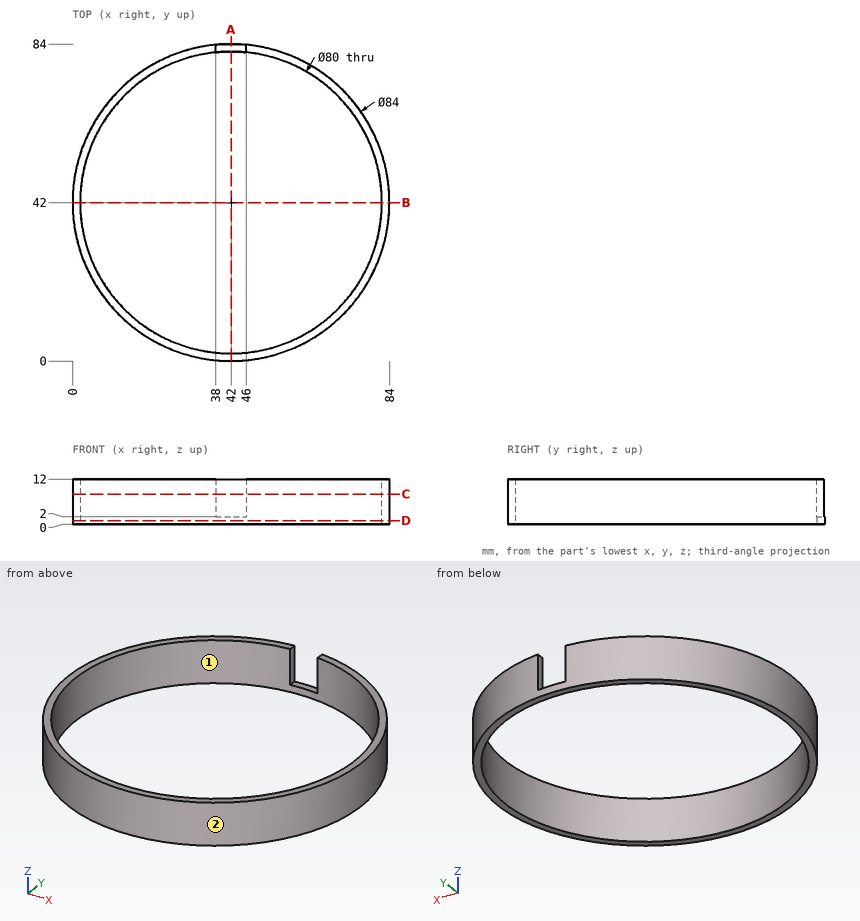
Drawing for the job (mm, zero at the part's lowest x, y, z). Give positions to 0.01 mm unless a question says otherwise; leave off trailing zeros. Order: outer loops, then holes, each group sorted by start corner. A loop starts at its lowest first (then second) coordinate and runs counter-clockwise, first axis right, second up. Notation, with made-up numbers: M -37.75,30.25 L -14.75,30.25 A17 cw -14.75,40.25 Z; hole C 56,-16.75 d10. An arc over 180 degrees is marked long. Write item = value, one per line. Start each with the question number.
(1) Slice it at A-A on x = 42. Write the cut outline in (y, z), plus the area to 3 significant figures.
(2) Slice it at C-C on z = 8. Write the cut outline in (x, y).
(3) Slice it at D-D on z = 1. Write the cut outline in (x, y).
(4) Two-plate mould, pull along X, no slides. Class the marked faces 1 and 2: released by +X, released by -X, zero draft, split by the parting line, or undercut.
(5) Probe L1, parallel to X at y = 42, z = 7.5; L2, parallel to Y at x = 42, z = 4; L3, parallel to Y at x = 52.5, z = 4.5. List the from-to ranges inside material, lowest first. Write a range as [from, to].
(6) Slice it at B-B on y = 42. Write the cut outline in (x, z).
(7) Pin check, flat tips, straight feed: pin 1 Ø5 at (y, z) = (31.5, 7.5) entering from -X; pin 2 Ø1.8 at (x, y) = (40.5, 83.5) entering from +Z; pin 3 Ø2 at (x, z) = (27.5, 9.5) entering from -Y; pin 4 Ø5 at (x, y) = (11, 10.5) entering from +Z. Stop position of each tip, or through.
Responses:
q1.outline = M 0,0 L 2,0 L 2,12 L 0,12 Z; M 82,0 L 84,0 L 84,2 L 82,2 Z
q1.area = 28.0 mm2
q2.outline = M 38,81.8 L 38,83.81 A42 ccw long 46,83.81 L 46,81.8 A40 cw long Z
q3.outline = C 42,42 d84; hole C 42,42 d80
q4.face_1 = undercut
q4.face_2 = split by the parting line
q5.L1 = [0, 2], [82, 84]
q5.L2 = [0, 2]
q5.L3 = [1.33, 3.4], [80.6, 82.67]
q6.outline = M 0,0 L 2,0 L 2,12 L 0,12 Z; M 82,0 L 84,0 L 84,12 L 82,12 Z
q7.pin_1 = 0.77
q7.pin_2 = 2
q7.pin_3 = 2.23
q7.pin_4 = 12
